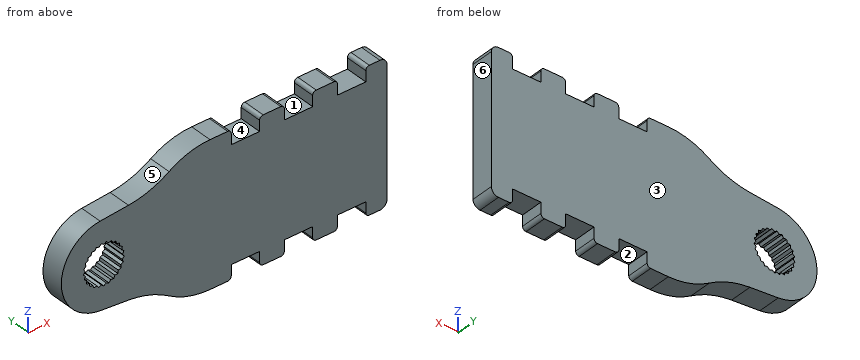
```python
from build123d import *

# Parameters (mm, degrees)
BOSS_EXTRUDE1_DEPTH = 3.175
FILLET2_R           = 1
FILLET3_R           = 0.5


with BuildPart() as part:
    # Sketch1 → Boss-Extrude1 (new body)
    with BuildSketch(Plane(origin=(0, 0, 0), x_dir=(1, 0, 0), z_dir=(0, 1, 0))):
        with BuildLine():
            Line((40, -10), (40, 10))
            Line((40, 10), (37, 10))
            Line((37, 10), (37, 8))
            Line((37, 8), (33, 8))
            Line((33, 8), (33, 10))
            Line((33, 10), (29.5, 10))
            Line((29.5, 10), (29.5, 8))
            Line((29.5, 8), (25.5, 8))
            Line((25.5, 8), (25.5, 10))
            Line((25.5, 10), (22, 10))
            Line((22, 10), (22, 8))
            Line((22, 8), (18, 8))
            Line((18, 8), (18, 10))
            Line((18, 10), (15, 10))
            ThreePointArc((15, 10), (11.981600452, 9.564316032), (9.209618064, 8.29283265))
            ThreePointArc((9.209618064, 8.29283265), (6.463385686, 6.959896642), (3.477065544, 6.327122843))
            Line((3.477065544, 6.327122843), (-0.522934456, 5.977168189))
            ThreePointArc((-0.522934456, 5.977168189), (-6, 0), (-0.522934456, -5.977168189))
            Line((-0.522934456, -5.977168189), (3.477065544, -6.327122843))
            ThreePointArc((3.477065544, -6.327122843), (6.463385686, -6.959896642), (9.209618064, -8.29283265))
            ThreePointArc((9.209618064, -8.29283265), (11.981600452, -9.564316032), (15, -10))
            Line((15, -10), (18, -10))
            Line((18, -10), (18, -8))
            Line((18, -8), (22, -8))
            Line((22, -8), (22, -10))
            Line((22, -10), (25.5, -10))
            Line((25.5, -10), (25.5, -8))
            Line((25.5, -8), (29.5, -8))
            Line((29.5, -8), (29.5, -10))
            Line((29.5, -10), (33, -10))
            Line((33, -10), (33, -8))
            Line((33, -8), (37, -8))
            Line((37, -8), (37, -10))
            Line((37, -10), (40, -10))
        make_face()
        Polygon((0, 2.895), (-0.332133069, 2.629103958), (-0.719957223, 2.804048251), (-0.975530065, 2.463907688), (-1.394676887, 2.536907839), (-1.557630919, 2.143895035), (-1.981763872, 2.110364176), (-2.041860093, 1.689173573), (-2.444329344, 1.551218571), (-2.397791689, 1.128315123), (-2.753308615, 0.894604199), (-2.603061214, 0.496560484), (-2.889287379, 0.181778554), (-2.64477083, -0.166394877), (-2.843721591, -0.542468906), (-2.520299768, -0.818895035), (-2.619474317, -1.232631049), (-2.237469003, -1.419941007), (-2.230635838, -1.84534245), (-1.814049831, -1.931766863), (-1.701638305, -2.342104199), (-1.276647236, -2.322212702), (-1.06572058, -2.691702927), (-0.659028201, -2.566745377), (-0.362839711, -2.87217206), (0, -2.65), (0.362839711, -2.87217206), (0.659028201, -2.566745377), (1.06572058, -2.691702927), (1.276647236, -2.322212702), (1.701638305, -2.342104199), (1.814049831, -1.931766863), (2.230635838, -1.84534245), (2.237469003, -1.419941007), (2.619474317, -1.232631049), (2.520299768, -0.818895035), (2.843721591, -0.542468906), (2.64477083, -0.166394877), (2.889287379, 0.181778554), (2.603061214, 0.496560484), (2.753308615, 0.894604199), (2.397791689, 1.128315123), (2.444329344, 1.551218571), (2.041860093, 1.689173573), (1.981763872, 2.110364176), (1.557630919, 2.143895035), (1.394676887, 2.536907839), (0.975530065, 2.463907688), (0.719957223, 2.804048251), (0.332133069, 2.629103958), align=None, mode=Mode.SUBTRACT)
    extrude(amount=BOSS_EXTRUDE1_DEPTH)

    # Fillet2
    fillet2_edges = [part.edges().sort_by_distance(p)[0] for p in [
        (40, 1.5875, -10),
        (40, 1.5875, 10),
    ]]
    fillet(fillet2_edges, radius=FILLET2_R)

    # Fillet3
    fillet3_edges = [part.edges().sort_by_distance(p)[0] for p in [
        (37, 1.5875, -10),
        (37, 1.5875, 10),
        (33, 1.5875, 10),
        (29.5, 1.5875, 10),
        (25.5, 1.5875, 10),
        (22, 1.5875, 10),
        (18, 1.5875, 10),
        (18, 1.5875, -10),
        (22, 1.5875, -10),
        (25.5, 1.5875, -10),
        (29.5, 1.5875, -10),
        (33, 1.5875, -10),
    ]]
    fillet(fillet3_edges, radius=FILLET3_R)


solid = part.part
```
Check sheet for the modelled part. Datum: model origin and axes. Units: mm. Face numbers are marked on the shaded views. A direction names the side the tool comes from. Round coordinates to 2 decimals unless told otherwise and drop trailing zeros. Loops run counter-clockwise (first coordinate to the right, second up) from the corner with the lowest first, then second, coordinate; pieces in that order, holes last. Notation, with made-up numbers: (27.25, 78.25) -> (66.25, 78.25) arc R27 ccw to (66.25, 95.25) -> close; hole circle Ø2 at (-5, 68). An arc over 180 degrees is marked (long way). Answer in a Markdown table with one row per item.
Q1. Release check for a two-part mould opening along X. For the marked faces 4, 5 and 6 record: released by +X, released by -X, zero draft, split by the parting line, or undercut.
Data:
| item | result |
|---|---|
| face 4 | undercut |
| face 5 | released by -X |
| face 6 | released by +X |
Q2. Sectioned sample at A-A on x = 34.5. Enter the section's corners in (y, z) (3 decimals).
Data:
| item | result |
|---|---|
| outline | (0, -8) -> (3.175, -8) -> (3.175, 8) -> (0, 8) -> close |
Q3. Sectioned sample at B-B on z = -4.5. Enter the section's corners in (x, y) (3 decimals).
Data:
| item | result |
|---|---|
| outline | (-3.969, 0) -> (40, 0) -> (40, 3.175) -> (-3.969, 3.175) -> close |
Q4. Set-up check for the marked faces 1, 2 and 3: record each of +Z, -Z, +X, -X, +Y, -Y from which the full face is reachable in a straight line by a thin tool's end or side.
Data:
| item | result |
|---|---|
| face 1 | +Z, +Y, -Y |
| face 2 | -Z, +Y, -Y |
| face 3 | +Z, -Z, +X, -X, +Y |
Q5. Thickness scan on L1, parallel to X at y = 0.1, z = 8.75; L2, parallel to Z at x = 27, y = 0.6; L3, parallel to Z at x = -1, y = 2. Record the ranges inside material, lowest first.
Data:
| item | result |
|---|---|
| L1 | x = 9.99 to 18, 22 to 25.5, 29.5 to 33, 37 to 40 |
| L2 | z = -8 to 8 |
| L3 | z = -5.92 to -2.47, 2.67 to 5.92 |
Q6. Go/stop test with flat-tipped pins: P1, Ø3, axis at x = 6.5, z = 7.5, coming from the -Y side; P2, Ø1.6, axis at x = 28, y = 1.5, coming from the -Z side; P3, Ø1.6, axis at y = 1, z = 8.5, coming from the -X side; P4, Ø1.6, axis at x = 27, y = 2, coming from the +Z side. Record where each tip stops, or that it passes through.
Data:
| item | result |
|---|---|
| P1 | stops at y = 0 |
| P2 | stops at z = -8 |
| P3 | stops at x = 8.19 |
| P4 | stops at z = 8 |
